CAD build for the part. Positions are in the model's coordinates, mm. Coordinates: 2 decimals unless noted, no trailing zeros. Order: outer loops, then holes, each group sorted by start corner. A loop starts at its lowest first (then second) coordinate and runs counter-clockwise, first axis right, second up. Notation, with made-up numbers: M 23.25,35.5 L 41.25,35.5 A24 cw 41.25,51.5 Z; hole C 71,-26 d8. An arc over 180 degrees is marked long. One line per item, written item: value.
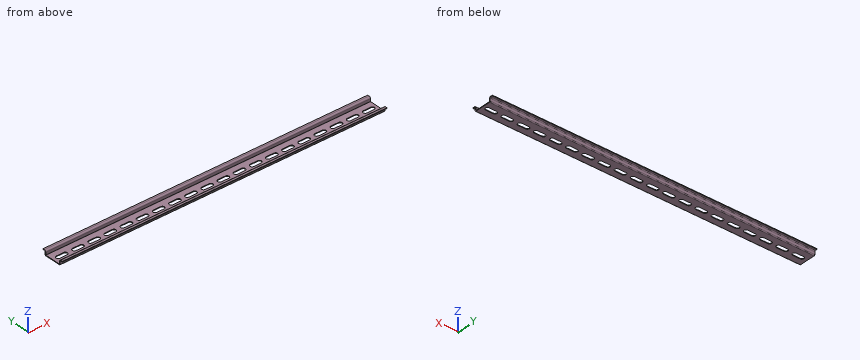
from build123d import *

# Parameters (mm, degrees)
STRUCTURAL_MEMBER1_DEPTH = 500
CUT_EXTRUDE1_REACH       = 252.724
LPATTERN1_DEPTH          = 1


# Read off the part's stored shape, not the designer's step: LPattern1
with BuildPart() as part:
    # Sketch2 → Structural Member1 (new body)
    with BuildSketch(Plane(origin=(-250, 0, 0), x_dir=(0, 0, -1), z_dir=(1, 0, 0))):
        with BuildLine():
            Line((0, 12.25), (0, -12.25))
            ThreePointArc((0, -12.25), (-0.366116524, -13.133883476), (-1.25, -13.5))
            Line((-1.25, -13.5), (-5.25, -13.5))
            ThreePointArc((-5.25, -13.5), (-6.133883476, -13.866116524), (-6.5, -14.75))
            Line((-6.5, -14.75), (-6.5, -17.5))
            Line((-6.5, -17.5), (-7.5, -17.5))
            Line((-7.5, -17.5), (-7.5, -14.75))
            ThreePointArc((-7.5, -14.75), (-6.840990258, -13.159009742), (-5.25, -12.5))
            Line((-5.25, -12.5), (-1.25, -12.5))
            ThreePointArc((-1.25, -12.5), (-1.073223305, -12.426776695), (-1, -12.25))
            Line((-1, -12.25), (-1, 12.25))
            ThreePointArc((-1, 12.25), (-1.073223305, 12.426776695), (-1.25, 12.5))
            Line((-1.25, 12.5), (-5.25, 12.5))
            ThreePointArc((-5.25, 12.5), (-6.840990258, 13.159009742), (-7.5, 14.75))
            Line((-7.5, 14.75), (-7.5, 17.5))
            Line((-7.5, 17.5), (-6.5, 17.5))
            Line((-6.5, 17.5), (-6.5, 14.75))
            ThreePointArc((-6.5, 14.75), (-6.133883476, 13.866116524), (-5.25, 13.5))
            Line((-5.25, 13.5), (-1.25, 13.5))
            ThreePointArc((-1.25, 13.5), (-0.366116524, 13.133883476), (0, 12.25))
        make_face()
    extrude(amount=STRUCTURAL_MEMBER1_DEPTH)

    # Sketch3 → Cut-Extrude1 (cut, up to next)
    with BuildSketch(Plane.XY, mode=Mode.PRIVATE) as cut_extrude1_sk1:
        with BuildLine():
            Line((-241.745, 3.175), (-230.315, 3.175))
            ThreePointArc((-230.315, 3.175), (-227.14, 0), (-230.315, -3.175))
            Line((-230.315, -3.175), (-241.745, -3.175))
            ThreePointArc((-241.745, -3.175), (-244.92, 0), (-241.745, 3.175))
        make_face()
    cut_extrude1_tool1 = extrude(cut_extrude1_sk1.sketch, amount=CUT_EXTRUDE1_REACH, mode=Mode.PRIVATE) & part.part
    add(cut_extrude1_tool1.solids().sort_by_distance((-236.03, 0, 0))[0], mode=Mode.SUBTRACT)

    # LPattern1 outline → LPattern1 (cut)
    with BuildSketch(Plane.XY):
        with BuildLine():
            Line((-216.853, -3.175), (-205.423, -3.175))
            ThreePointArc((-205.423, -3.175), (-202.248, 0), (-205.423, 3.175))
            Line((-205.423, 3.175), (-216.853, 3.175))
            ThreePointArc((-216.853, 3.175), (-220.028, 0), (-216.853, -3.175))
        make_face()
        with BuildLine():
            Line((-191.961, -3.175), (-180.531, -3.175))
            ThreePointArc((-180.531, -3.175), (-177.356, 0), (-180.531, 3.175))
            Line((-180.531, 3.175), (-191.961, 3.175))
            ThreePointArc((-191.961, 3.175), (-195.136, 0), (-191.961, -3.175))
        make_face()
        with BuildLine():
            Line((-167.069, -3.175), (-155.639, -3.175))
            ThreePointArc((-155.639, -3.175), (-152.464, 0), (-155.639, 3.175))
            Line((-155.639, 3.175), (-167.069, 3.175))
            ThreePointArc((-167.069, 3.175), (-170.244, 0), (-167.069, -3.175))
        make_face()
        with BuildLine():
            Line((-142.177, -3.175), (-130.747, -3.175))
            ThreePointArc((-130.747, -3.175), (-127.572, 0), (-130.747, 3.175))
            Line((-130.747, 3.175), (-142.177, 3.175))
            ThreePointArc((-142.177, 3.175), (-145.352, 0), (-142.177, -3.175))
        make_face()
        with BuildLine():
            Line((-117.285, -3.175), (-105.855, -3.175))
            ThreePointArc((-105.855, -3.175), (-102.68, 0), (-105.855, 3.175))
            Line((-105.855, 3.175), (-117.285, 3.175))
            ThreePointArc((-117.285, 3.175), (-120.46, 0), (-117.285, -3.175))
        make_face()
        with BuildLine():
            Line((-92.393, -3.175), (-80.963, -3.175))
            ThreePointArc((-80.963, -3.175), (-77.788, 0), (-80.963, 3.175))
            Line((-80.963, 3.175), (-92.393, 3.175))
            ThreePointArc((-92.393, 3.175), (-95.568, 0), (-92.393, -3.175))
        make_face()
        with BuildLine():
            Line((-67.501, -3.175), (-56.071, -3.175))
            ThreePointArc((-56.071, -3.175), (-52.896, 0), (-56.071, 3.175))
            Line((-56.071, 3.175), (-67.501, 3.175))
            ThreePointArc((-67.501, 3.175), (-70.676, 0), (-67.501, -3.175))
        make_face()
        with BuildLine():
            Line((-42.609, -3.175), (-31.179, -3.175))
            ThreePointArc((-31.179, -3.175), (-28.004, 0), (-31.179, 3.175))
            Line((-31.179, 3.175), (-42.609, 3.175))
            ThreePointArc((-42.609, 3.175), (-45.784, 0), (-42.609, -3.175))
        make_face()
        with BuildLine():
            Line((-17.717, -3.175), (-6.287, -3.175))
            ThreePointArc((-6.287, -3.175), (-3.112, 0), (-6.287, 3.175))
            Line((-6.287, 3.175), (-17.717, 3.175))
            ThreePointArc((-17.717, 3.175), (-20.892, 0), (-17.717, -3.175))
        make_face()
        with BuildLine():
            Line((7.175, -3.175), (18.605, -3.175))
            ThreePointArc((18.605, -3.175), (21.78, 0), (18.605, 3.175))
            Line((18.605, 3.175), (7.175, 3.175))
            ThreePointArc((7.175, 3.175), (4, 0), (7.175, -3.175))
        make_face()
        with BuildLine():
            Line((32.067, -3.175), (43.497, -3.175))
            ThreePointArc((43.497, -3.175), (46.672, 0), (43.497, 3.175))
            Line((43.497, 3.175), (32.067, 3.175))
            ThreePointArc((32.067, 3.175), (28.892, 0), (32.067, -3.175))
        make_face()
        with BuildLine():
            Line((56.959, -3.175), (68.389, -3.175))
            ThreePointArc((68.389, -3.175), (71.564, 0), (68.389, 3.175))
            Line((68.389, 3.175), (56.959, 3.175))
            ThreePointArc((56.959, 3.175), (53.784, 0), (56.959, -3.175))
        make_face()
        with BuildLine():
            Line((81.851, -3.175), (93.281, -3.175))
            ThreePointArc((93.281, -3.175), (96.456, 0), (93.281, 3.175))
            Line((93.281, 3.175), (81.851, 3.175))
            ThreePointArc((81.851, 3.175), (78.676, 0), (81.851, -3.175))
        make_face()
        with BuildLine():
            Line((106.743, -3.175), (118.173, -3.175))
            ThreePointArc((118.173, -3.175), (121.348, 0), (118.173, 3.175))
            Line((118.173, 3.175), (106.743, 3.175))
            ThreePointArc((106.743, 3.175), (103.568, 0), (106.743, -3.175))
        make_face()
        with BuildLine():
            Line((131.635, -3.175), (143.065, -3.175))
            ThreePointArc((143.065, -3.175), (146.24, 0), (143.065, 3.175))
            Line((143.065, 3.175), (131.635, 3.175))
            ThreePointArc((131.635, 3.175), (128.46, 0), (131.635, -3.175))
        make_face()
        with BuildLine():
            Line((156.527, -3.175), (167.957, -3.175))
            ThreePointArc((167.957, -3.175), (171.132, 0), (167.957, 3.175))
            Line((167.957, 3.175), (156.527, 3.175))
            ThreePointArc((156.527, 3.175), (153.352, 0), (156.527, -3.175))
        make_face()
        with BuildLine():
            Line((181.419, -3.175), (192.849, -3.175))
            ThreePointArc((192.849, -3.175), (196.024, 0), (192.849, 3.175))
            Line((192.849, 3.175), (181.419, 3.175))
            ThreePointArc((181.419, 3.175), (178.244, 0), (181.419, -3.175))
        make_face()
        with BuildLine():
            Line((206.311, -3.175), (217.741, -3.175))
            ThreePointArc((217.741, -3.175), (220.916, 0), (217.741, 3.175))
            Line((217.741, 3.175), (206.311, 3.175))
            ThreePointArc((206.311, 3.175), (203.136, 0), (206.311, -3.175))
        make_face()
        with BuildLine():
            Line((231.203, -3.175), (242.633, -3.175))
            ThreePointArc((242.633, -3.175), (245.808, 0), (242.633, 3.175))
            Line((242.633, 3.175), (231.203, 3.175))
            ThreePointArc((231.203, 3.175), (228.028, 0), (231.203, -3.175))
        make_face()
    extrude(amount=LPATTERN1_DEPTH, mode=Mode.SUBTRACT)


solid = part.part
Q1. Drill centre lines: line 1 along Y through (x, z) = (-12, 4.5); line 2 along Z through (x, y) = (77, -11); line 3 along Y through (x, z) = (66, 6.75). Where is each one in solid material? Low to high.
Recorded:
line 1: y = -13.5 to -12.5, 12.5 to 13.5
line 2: z = 0 to 1
line 3: y = -17.5 to -13.07, 13.07 to 17.5
Q2. Slice it at A-A (z = 4). List the corners of the cut face in (x, y).
Recorded:
outline: M -250,-13.5 L 250,-13.5 L 250,-12.5 L -250,-12.5 Z; M -250,12.5 L 250,12.5 L 250,13.5 L -250,13.5 Z
Q3. Pin check, flat tips, straight feed: pin 1 Ø6 at (x, y) = (-71.5, -2.5) entering from -Z; pin 2 Ø0.8 at (x, z) = (160, 0.5) entering from -Y; pin 3 Ø1.1 at (x, z) = (-9.5, 0.5) entering from +Y; pin 4 Ø19.5 at (x, y) = (56.5, 0.5) entering from +Z. Stop position of each tip, or through.
Recorded:
pin 1: stops at z = 0
pin 2: stops at y = -13.45
pin 3: stops at y = 13.48
pin 4: stops at z = 1
